Can you work these out from the model? Positions are in its coordinate system, mm. Face numbers are marked on the shaded views. A direction names the side the tool comes from. Give positions to 0.01 mm unless a question says otherwise; leave off trailing zeros. Order: outer loops, then holes, each group sorted by start corner. A loop starts at its lowest first (then second) coordinate and runs counter-clockwise, first axis right, second up.
Item 1: I want a section at C-C, the plane z = 0. Write out the boundary of the cut face in (x, y), then the cut area to 3 significant figures.
Item 2: If we mould it in two halves opening along Y, with no side actions, what happens to the marked faces 1, 2 and 3? For each: +Y half, -Y half, draft (parallel to the pull), parting line (faces both ways), or undercut.
Item 3: If I drill on line 1 along X through (y, z) = (-2.45, 2.5); line 2 along Z through (x, y) = (-0.1, 2.7); line 3 along X through (y, z) = (2.4, 3.75), over which ranges is the centre line in solid material (lowest first)?
Item 4: I'm going to push flat-ended pins straight in: pin 1 Ø0.6 at (y, z) = (2.5, 4) entering from +X; pin 2 Ø1 at (x, y) = (-0.5, -1) entering from +Z; pin 3 Ø2 at (x, z) = (2.5, -0.5) entering from +Y; pin 4 Ø1.8 at (x, y) = (1, -1.5) entering from -Z. Where does each tip first touch, or does it pass through?
Item 5: Which directions (+Z, -Z, +X, -X, +Y, -Y) give clear straight access to the entire face, cutting with the end or side of a thin tool? Please do the marked faces 4 and 5.
Item 6: I want a section at B-B, the plane y = 2.35. Write out the boundary of the cut face in (x, z).
Item 7: I want a section at D-D, the plane x = 0.8. Write out the boundary of the cut face in (y, z), then the cut area to 3 significant figures.
Item 8: I want a section at A-A, the plane z = 3.75. Write out the boundary of the cut face in (x, y).
```python
from build123d import *

# Parameters (mm, degrees)
F0_W     = 6
F0_H     = 6
F1_DEPTH = 1.75
F2_R     = 1.75
F3_DEPTH = 1.5
F4_R     = 0.2
F6_DEPTH = 1.5


# Not quite as in the source:
# - a pattern or mirror of a feature is missing from the dataset's text; its kind, count and spacing are read off the source's solid


with BuildPart() as f1:
    # F0 (on Right) → F1 (new body, symmetric)
    with BuildSketch(Plane.YZ):
        Rectangle(F0_W, F0_H)
    extrude(amount=F1_DEPTH, both=True)

    # F2 (on face) → F3 (join)
    with BuildSketch(Plane.YZ.offset(1.75)):
        Circle(F2_R)
    extrude(amount=F3_DEPTH)

    # F4
    f4_edges = [f1.edges().sort_by_distance(p)[0] for p in [
        (3.25, -1.75, 0),
        (0, -3, 3),
        (0, 3, 3),
        (0, 3, -3),
        (0, -3, -3),
    ]]
    fillet(f4_edges, radius=F4_R)

    # F5 (on face) → F6 (join)
    with BuildSketch(Plane.XY.offset(3)):
        with BuildLine():
            ThreePointArc((-1.55, -2.7), (-1.5207106781, -2.7707106781), (-1.45, -2.8))
            Line((-1.45, -2.8), (-0.75, -2.8))
            ThreePointArc((-0.75, -2.8), (-0.6792893219, -2.7707106781), (-0.65, -2.7))
            Line((-0.65, -2.7), (-0.65, -2))
            ThreePointArc((-0.65, -2), (-0.6792893219, -1.9292893219), (-0.75, -1.9))
            Line((-0.75, -1.9), (-1.45, -1.9))
            ThreePointArc((-1.45, -1.9), (-1.5207106781, -1.9292893219), (-1.55, -2))
            Line((-1.55, -2), (-1.55, -2.7))
        make_face()
        with BuildLine():
            ThreePointArc((-0.65, 2.7), (-0.6792893219, 2.7707106781), (-0.75, 2.8))
            Line((-0.75, 2.8), (-1.45, 2.8))
            ThreePointArc((-1.45, 2.8), (-1.5207106781, 2.7707106781), (-1.55, 2.7))
            Line((-1.55, 2.7), (-1.55, 2))
            ThreePointArc((-1.55, 2), (-1.5207106781, 1.9292893219), (-1.45, 1.9))
            Line((-1.45, 1.9), (-0.75, 1.9))
            ThreePointArc((-0.75, 1.9), (-0.6792893219, 1.9292893219), (-0.65, 2))
            Line((-0.65, 2), (-0.65, 2.7))
        make_face()
    f6 = extrude(amount=F6_DEPTH)

    # F6_copies: F6 across plane
    add(f6.mirror(Plane(origin=(0, 0, 0), x_dir=(-1, 0, 0), z_dir=(0, 0, -1))))


solid = f1.part
```
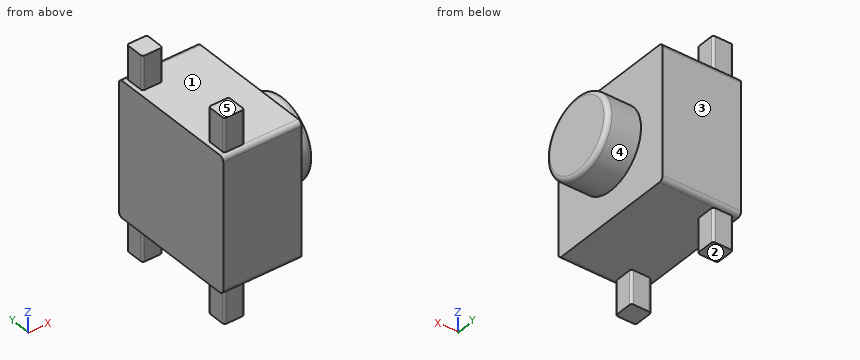
Results list:
1. outline: (-1.75, -3) - (1.75, -3) - (1.75, -1.75) - (3.05, -1.75) arc R0.2 ccw to (3.25, -1.55) - (3.25, 1.55) arc R0.2 ccw to (3.05, 1.75) - (1.75, 1.75) - (1.75, 3) - (-1.75, 3) - close
1. area: 26.2 mm2
2. face 1: undercut
2. face 2: draft
2. face 3: +Y half
3. line 1: x = -1.75 to 1.75
3. line 2: z = -3 to 3
3. line 3: x = -1.55 to -0.65
4. pin 1: stops at x = -0.65
4. pin 2: stops at z = 3
4. pin 3: stops at y = 3
4. pin 4: stops at z = -3
5. face 4: +X
5. face 5: +Z, +X, -X, +Y, -Y
6. outline: (-1.75, -3) - (-1.55, -3) - (-1.55, -4.5) - (-0.65, -4.5) - (-0.65, -3) - (1.75, -3) - (1.75, 3) - (-0.65, 3) - (-0.65, 4.5) - (-1.55, 4.5) - (-1.55, 3) - (-1.75, 3) - close
7. outline: (-3, -2.8) arc R0.2 ccw to (-2.8, -3) - (2.8, -3) arc R0.2 ccw to (3, -2.8) - (3, 2.8) arc R0.2 ccw to (2.8, 3) - (-2.8, 3) arc R0.2 ccw to (-3, 2.8) - close
7. area: 36.0 mm2
8. outline: (-1.55, -2.7) arc R0.1 ccw to (-1.45, -2.8) - (-0.75, -2.8) arc R0.1 ccw to (-0.65, -2.7) - (-0.65, -2) arc R0.1 ccw to (-0.75, -1.9) - (-1.45, -1.9) arc R0.1 ccw to (-1.55, -2) - close; (-1.55, 2) arc R0.1 ccw to (-1.45, 1.9) - (-0.75, 1.9) arc R0.1 ccw to (-0.65, 2) - (-0.65, 2.7) arc R0.1 ccw to (-0.75, 2.8) - (-1.45, 2.8) arc R0.1 ccw to (-1.55, 2.7) - close
